```python
from build123d import *

# Parameters (mm, degrees)
F0_R     = 12
F1_DEPTH = 2
F2_R     = 8.9467567694
F3_DEPTH = 5
F4_R     = 4.7902731663
F5_DEPTH = 3


# Not quite as in the source:
# - a fillet or chamfer that OpenCascade refuses, or shapes differently, is made with other operations: its cross-section is extruded or revolved along the edge and cut away or added


with BuildPart() as f1:
    # F0 (on Top) → F1 (new body)
    with BuildSketch(Plane.XY):
        Circle(F0_R)
    extrude(amount=F1_DEPTH)

    # F2 (on face) → F3 (join)
    with BuildSketch(Plane.XY.offset(2)):
        Circle(F2_R)
    extrude(amount=F3_DEPTH)

    # F4 (on face) → F5 (cut)
    with BuildSketch(Plane.XY.offset(7)):
        Circle(F4_R)
    extrude(amount=-F5_DEPTH, mode=Mode.SUBTRACT)

    # F6: fillet of radius 5 on 1 edges, made by hand

    # F6_s1 → F6_t2 (revolve, cut)
    with BuildSketch(Plane.XZ):
        with BuildLine():
            ThreePointArc((12, 2), (10.2360679775, 0.527864045), (8, 0))
            Line((8, 0), (12, 0))
            Line((12, 0), (12, 2))
        make_face()
    revolve(axis=Axis((0, 0, 0), (0, 0, 1)), mode=Mode.SUBTRACT)


solid = f1.part
```
Geometry check sheet. Reference: the model listing, model coordinates, mm. A direction names the side the tool comes from. Coordinates: 2 decimals unless noted, no trailing zeros. Order: outer loops, then holes, each group sorted by start corner. A loop starts at its lowest first (then second) coordinate and runs counter-clockwise, first axis right, second up.
Q1. Depth check by flat-ended pin: pin 1 Ø1 at (y, z) = (-1, 6) entering from -X. Enter the tip coordinate at first touch or a pass-through.
Reply:
pin 1: stops at x = -8.93
Q2. Tool access check on faces 4 (the face through (4.57, 1.44, 5.52)), 5 (the face through (0, 0, 0)). Record the directions out of +Z, -Z, +X, -X, +Y, -Y that give a thin tool (end or side, any length) a straight path to the whole face; none if there is none.
Reply:
face 4: +Z
face 5: -Z, +X, -X, +Y, -Y
Q3. Sectioned sample at C-C on z = 5.5. Record the cut outline in (x, y), and give its area (3 significant figures).
Reply:
outline: circle Ø17.89 at (0, 0); hole circle Ø9.58 at (0, 0)
area: 179 mm2
Q4. Sectioned sample at A-A on x = 0. Record the cut outline in (y, z), and give its area (3 significant figures).
Reply:
outline: (-12, 2) arc R5 ccw to (-8, 0) - (8, 0) arc R5 ccw to (12, 2) - (8.95, 2) - (8.95, 7) - (4.79, 7) - (4.79, 4) - (-4.79, 4) - (-4.79, 7) - (-8.95, 7) - (-8.95, 2) - close
area: 104 mm2
Q5. Draft check along Y on faces 1 (the face through (-5, -8, 2)), 2 (the face through (4.128, -7.937, 4.465)), 3 (the face through (0, 0, 4)). Enter one of: released by +Y, released by -Y, zero draft, split by the parting line, or undercut.
Reply:
face 1: zero draft
face 2: split by the parting line
face 3: undercut
Q6. Sectioned sample at D-D on z = 3.5. Record the cut outline in (x, y).
Reply:
outline: circle Ø17.89 at (0, 0)
Q7. Thickness scan on probe 1 along Y at (x, z) = (0, 5.55); probe 2 along Z at (x, y) = (0, -8.25); probe 3 along Y at (x, z) = (3.5, 6.5). Record the ranges inside material, lowest first.
Reply:
probe 1: y = -8.95 to -4.79, 4.79 to 8.95
probe 2: z = 0.01 to 7
probe 3: y = -8.23 to -3.27, 3.27 to 8.23
